Part print with two shaded views. Sizes in mm from the minimum x, y, z corner. A direction names the side the tool comes from. Coordinates: 2 decimals unless noted, no trailing zeros. Order: outer loops, then holes, each group sorted by start corner. A loop starts at its lowest first (then second) coordinate and runs counter-clockwise, first axis right, second up.
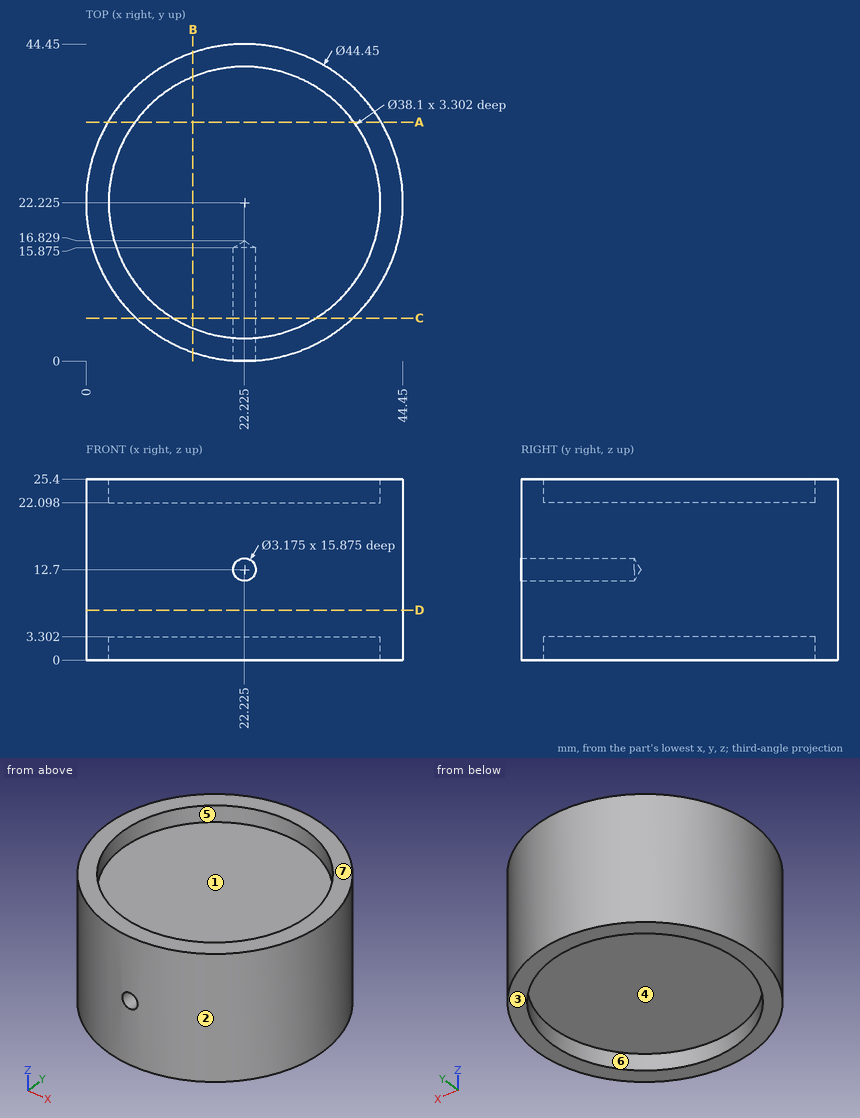
Q1. Cut at A-A on y = 33.5. Write the cut outline in (x, z).
Results list:
outline: (3.07, 0) - (6.87, 0) - (6.87, 3.3) - (37.58, 3.3) - (37.58, 0) - (41.38, 0) - (41.38, 25.4) - (37.58, 25.4) - (37.58, 22.1) - (6.87, 22.1) - (6.87, 25.4) - (3.07, 25.4) - close
Q2. Which spindle directions (+Z, -Z, +X, -X, +Y, -Y) get a long thin tool onto all of the face, cutting with end or side? Do the marked faces 5, 6 and 7. Say none if no direction does.
Results list:
face 5: +Z
face 6: -Z
face 7: +Z, +X, -X, +Y, -Y
Q3. Mould opens along X. For the marked faces 1, 2, 3 and 4 say: pulls with the +X half, pulls with the -X half, needs draft (parallel to the pull), parting line crosses it, or undercut.
Results list:
face 1: undercut
face 2: parting line crosses it
face 3: needs draft
face 4: undercut
Q4. Cut at D-D on z = 7. Write the cut outline in (x, y) (3 decimals).
Results list:
outline: circle Ø44.45 at (22.225, 22.225)
Q5. Pin check, flat tips, straight feed: pin 1 Ø10 at (y, z) = (21.5, 4.5) entering from +X; pin 2 Ø2 at (y, z) = (38.5, 7) entering from +X; pin 3 Ø2 at (y, z) = (20.5, 22) entering from -X. Stop position of each tip, or through.
Results list:
pin 1: stops at x = 44.45
pin 2: stops at x = 38.37
pin 3: stops at x = 0.01
Q6. Cut at C-C on y = 6. Write the cut outline in (x, z) (1 decimal).
Results list:
outline: (7, 0) - (12.2, 0) - (12.2, 3.3) - (32.2, 3.3) - (32.2, 0) - (37.4, 0) - (37.4, 25.4) - (32.2, 25.4) - (32.2, 22.1) - (12.2, 22.1) - (12.2, 25.4) - (7, 25.4) - close; hole circle Ø3.2 at (22.2, 12.7)
Q7. Cut at B-B on x = 15. Write the cut outline in (y, z), and give its area (3 significant figures).
Results list:
outline: (1.21, 0) - (4.6, 0) - (4.6, 3.3) - (39.85, 3.3) - (39.85, 0) - (43.24, 0) - (43.24, 25.4) - (39.85, 25.4) - (39.85, 22.1) - (4.6, 22.1) - (4.6, 25.4) - (1.21, 25.4) - close
area: 835 mm2
Q8. Wall check: line 1 along Y through (x, z) = (28, 2.25); line 2 along X through (y, z) = (26.5, 1.75) (1 decimal); line 3 along Y through (x, z) = (6.5, 2.25). Give the ranges that are in metal, low to high.
Results list:
line 1: y = 0.76 to 4.07, 40.38 to 43.69
line 2: x = 0.4 to 3.7, 40.8 to 44
line 3: y = 6.52 to 11.47, 32.98 to 37.93
